```python
from build123d import *

# Parameters (mm, degrees)
F2_R     = 0.25
F3_SIZE  = 0.3
F4_SIZE2 = 2.5
F4_SIZE  = 0.5


with BuildPart() as f1:
    # F0 (on Right) → F1 (revolve)
    with BuildSketch(Plane.YZ):
        Polygon((0, 9.95), (0, 2.5), (10, 2.5), (10, 6), (2.8, 6), (2.8, 9.95), align=None)
    revolve(axis=Axis((0, 5.3417352028, 0), (0, 1, 0)))

    # F2
    f2_edges = [f1.edges().sort_by_distance(p)[0] for p in [
        (0, 2.8, -6),
    ]]
    fillet(f2_edges, radius=F2_R)

    # F3
    f3_edges = [f1.edges().sort_by_distance(p)[0] for p in [
        (0, 10, -6),
    ]]
    chamfer(f3_edges, length=F3_SIZE)

    # F4
    f4_edges = [f1.edges().sort_by_distance(p)[0] for p in [
        (0, 0, -9.95),
        (0, 2.8, -9.95),
    ]]
    f4_side = f1.faces().sort_by_distance((0, 1.4, -9.95))[0]
    chamfer(f4_edges, length=F4_SIZE, length2=F4_SIZE2, reference=f4_side)


solid = f1.part
```
Verification items for the finished model (mm, model axes). A direction names the side the tool comes from. Coordinates: 2 decimals unless noted, no trailing zeros. Loops run counter-clockwise (first coordinate to the right, second up) from the corner with the lowest first, then second, coordinate; pieces in that order, holes last. Notation, with made-up numbers: (63.5, 42) -> (104.5, 42) arc R29 ccw to (104.5, 63) -> close; hole circle Ø6 at (47.25, -30.5). An arc over 180 degrees is marked (long way). Answer in a Markdown table with one row per item. Add a question column.
1. Access from +Z, -Z, +X, -X, +Y, -Y to the whole of each face (thin tool, end or side, straight path). Record for faces 4 (the face through (0, 6, -6)), 5 (the face through (0, 0, 3)).
2. Material ranges on probe 1 along X at (y, z) = (6.75, 0); probe 2 along Z at (x, y) = (1.75, 3.25); probe 3 along Z at (x, y) = (1, 0.75), recorded low to high. Write a range as [from, to].
3. Section check A-A, the plane z = 0. Enter the section's corners in (x, y), then the cut area to 3 significant figures.
4. Section check B-B, the plane y = 7.5. Enter the section's corners in (x, z), then the cut area to 3 significant figures.
5. Depth check by flat-ended pin: P1, Ø2, axis at y = 5, z = -1, coming from the +X side; P2, Ø6, axis at y = 6.5, z = -1.5, coming from the -X side; P3, Ø6, axis at y = 3.5, z = -5, coming from the +X side. Enter the tip coordinate at first touch or a pass-through.
6. Draft check along Z on faces 1 (the face through (-2.44, 5.07, -0.54)), 2 (the face through (-6.05, 1.39, -7.9)), 3 (the face through (-2.5, 10, -1.2)). Enter one of: +Z half, -Z half, draft (parallel to the pull), parting line (faces both ways), or undercut.
Derived:
| question | item | result |
|---|---|---|
| 1 | face 4 | +Y |
| 1 | face 5 | +Z, -Z, +X, -X, -Y |
| 2 | probe 1 | x = [-6, -2.5], [2.5, 6] |
| 2 | probe 2 | z = [-5.74, -1.79], [1.79, 5.74] |
| 2 | probe 3 | z = [-9.9, -2.29], [2.29, 9.9] |
| 3 | outline | (-9.95, 0.5) -> (-7.45, 0) -> (-2.5, 0) -> (-2.5, 10) -> (-5.7, 10) -> (-6, 9.7) -> (-6, 3.05) arc R0.25 cw to (-6.25, 2.8) -> (-7.45, 2.8) -> (-9.95, 2.3) -> close; (2.5, 0) -> (7.45, 0) -> (9.95, 0.5) -> (9.95, 2.3) -> (7.45, 2.8) -> (6.25, 2.8) arc R0.25 cw to (6, 3.05) -> (6, 9.7) -> (5.7, 10) -> (2.5, 10) -> close |
| 3 | area | 89.6 mm² |
| 4 | outline | circle Ø12 at (0, 0); hole circle Ø5 at (0, 0) |
| 4 | area | 93.5 mm² |
| 5 | P1 | stops at x = 6 |
| 5 | P2 | stops at x = -6 |
| 5 | P3 | stops at x = 9.69 |
| 6 | face 1 | undercut |
| 6 | face 2 | parting line |
| 6 | face 3 | draft |
